Input: part model. Units: mm. Frame: model coordinates. Face numbers are marked on the shaded views. A direction names the side the tool comes from. Give positions to 0.01 mm unless a question says otherwise; leave off trailing zeros. Loops run counter-clockwise (first coordinate to the right, second up) from the corner with the lowest first, then second, coordinate; pieces in that order, holes last. Notation, with made-up numbers: (-9, 32) - (42, 32) arc R26 cw to (42, 60) - close; hole circle Ø3 at (33, -13.5). An arc over 180 degrees is marked (long way). Answer as a JSON object with one key per item and string values. Group by question number.
(1) Section query C-C (x = 0.85). Return loops of the section in (y, z), plus the area to 3 significant figures.
(2) Mould query, pull axis X, two halves, no side actions, for the marked faces 1, 2 and 3. Classes: +X half, -X half, draft (parallel to the pull), parting line (faces both ways), or undercut.
(3) Access query for the marked faces 4 and 5. Directions: +Z, -Z, +X, -X, +Y, -Y. A direction counts if a zero-diameter tool reaches every point of the face in a straight line with its end or side. Return the directions, or none.
(4) Section query D-D (x = 1.7). Return loops of the section in (y, z), plus the area to 3 significant figures.
(5) Pin query (flat end, axial travel): P1, Ø1, axis at y = -0.5, z = 15.5, coming from the -X side; P2, Ø1.5, axis at x = -1.5, z = 4.5, coming from the +Y side; P3, Ø1.5, axis at x = -0.5, y = 0.5, coming from the -Z side. Return the tip coordinate at first contact, or that it passes through.
(6) Section query B-B (z = 11.75). Return loops of the section in (x, y), plus the area to 3 significant figures.
(7) Section query A-A (y = 0). Return loops of the section in (x, z).
(8) Material intervals for L1, parallel to Z at x = -1.75, y = 2; L2, parallel to Z at x = -0.85, y = 0.9; L3, parallel to X at y = -1.9, z = 1.75, sorted ascending.
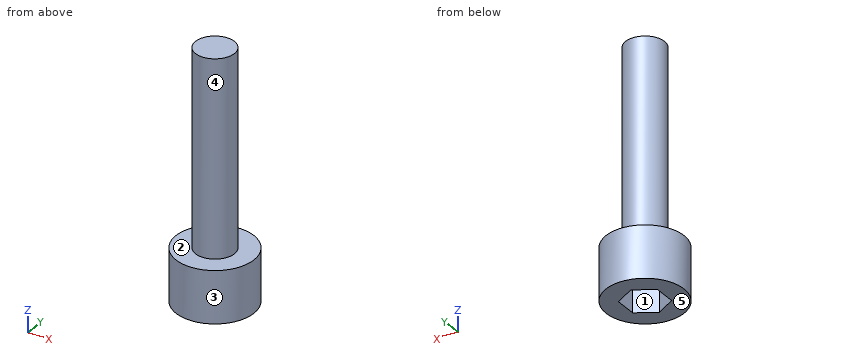
Solid Edge part; units mm, degrees
sketch "Sketch1" plane through (0, 0, 0) normal (0, 0, 1) x (1, 0, 0)
  circle A0 centre (0, 0) radius 3
extrude "Protrusion1" add sketch "Sketch1" along normal blind 4
sketch "Sketch2" plane through (0, 0, 4) normal (0, 0, 1) x (1, 0, 0)
  circle A0 centre (0, 0) radius 1.5
extrude "Bult" add sketch "Sketch2" along normal blind 15
sketch "Sketch3" plane through (0, 0, 0) normal (0, 0, -1) x (1, 0, 0)
  line L0 (1.5, 0.866) -> (0, 1.7321)
  line L1 (0, 1.7321) -> (-1.5, 0.866)
  line L2 (-1.5, 0.866) -> (-1.5, -0.866)
  line L3 (-1.5, -0.866) -> (0, -1.7321)
  line L4 (0, -1.7321) -> (1.5, -0.866)
  line L5 (1.5, -0.866) -> (1.5, 0.866)
  dimension "D1" = 1.5
  dimension "D2" = 1.5
extrude "Försänkning_skruv" cut sketch "Sketch3" against normal blind 2.5
Recorded:
{
 "1": {"outline": "(-2.88, 0) - (-1.24, 0) - (-1.24, 2.5) - (1.24, 2.5) - (1.24, 0) - (2.88, 0) - (2.88, 4) - (1.24, 4) - (1.24, 19) - (-1.24, 19) - (-1.24, 4) - (-2.88, 4) - close", "area": "53.9 mm^2"},
 "2": {"face 1": "undercut", "face 2": "draft", "face 3": "parting line"},
 "3": {"face 4": "+Z", "face 5": "-Z, +X, -X, +Y, -Y"},
 "4": {"outline": "(-2.47, 0) - (2.47, 0) - (2.47, 4) - (-2.47, 4) - close", "area": "19.8 mm^2"},
 "5": {"P1": "stops at x = -1.5", "P2": "stops at y = 2.85", "P3": "stops at z = 2.5"},
 "6": {"outline": "circle Ø3 at (0, 0)", "area": "7.07 mm^2"},
 "7": {"outline": "(-3, 0) - (-1.5, 0) - (-1.5, 2.5) - (1.5, 2.5) - (1.5, 0) - (3, 0) - (3, 4) - (1.5, 4) - (1.5, 19) - (-1.5, 19) - (-1.5, 4) - (-3, 4) - close"},
 "8": {"L1": "z = 0 to 4", "L2": "z = 2.5 to 19", "L3": "x = -2.32 to 2.32"}
}
